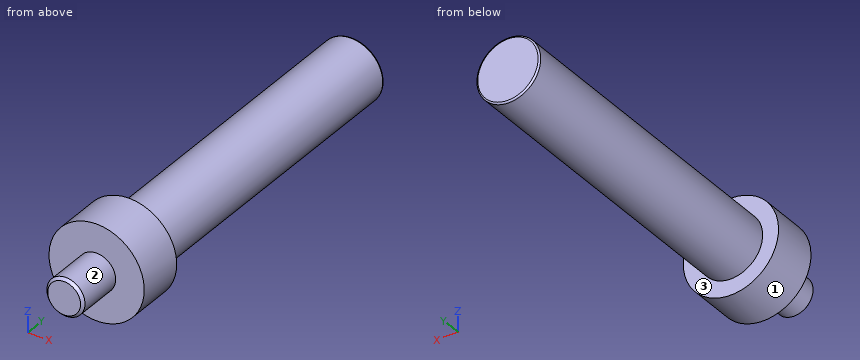
```python
from build123d import *

# Parameters (mm, degrees)
SKETCH1_R           = 15
BOSS_EXTRUDE1_DEPTH = 15
SKETCH2_R           = 10
BOSS_EXTRUDE2_DEPTH = 103
SKETCH3_R           = 7.5
BOSS_EXTRUDE3_DEPTH = 15
FILLET1_R           = 0.5


# Read off the part's stored shape, not the designer's step: M12x1.5 Machine Threads Stud1
with BuildPart() as part:
    # Sketch1 → Boss-Extrude1 (new body)
    with BuildSketch(Plane(origin=(0, 0, 0), x_dir=(1, 0, 0), z_dir=(0, 1, 0))):
        with Locations(Location((0, 0, 0), (0, 0, 270))):
            Circle(SKETCH1_R)
    extrude(amount=BOSS_EXTRUDE1_DEPTH)

    # Sketch2 → Boss-Extrude2 (add)
    with BuildSketch(Plane(origin=(0, 15, 0), x_dir=(1, 0, 0), z_dir=(0, 1, 0))):
        with Locations(Location((0, 0, 0), (0, 0, 270))):
            Circle(SKETCH2_R)
    extrude(amount=BOSS_EXTRUDE2_DEPTH)

    # Sketch3 → Boss-Extrude3 (add)
    with BuildSketch(Plane.XZ):
        with Locations(Location((0, 0, 0), (0, 0, 270))):
            Circle(SKETCH3_R)
    extrude(amount=BOSS_EXTRUDE3_DEPTH)

    # M12x1.5 Machine Threads Stud1 outline → M12x1.5 Machine Threads Stud1 (revolve, cut)
    with BuildSketch(Plane.XY):
        Polygon((7.5, 0), (6, 0), (6, -14.172), (5.172, -15), (7.5, -15), align=None)
    revolve(axis=Axis((0, 0, 0), (0, 1, 0)), mode=Mode.SUBTRACT)

    # Fillet1
    fillet1_edges = [part.edges().sort_by_distance(p)[0] for p in [
        (0, 118, -10),
    ]]
    fillet(fillet1_edges, radius=FILLET1_R)


solid = part.part
```
Build history of the part. All positions in model axes, mm. Face numbers are marked on the shaded views. A direction names the side the tool comes from. Round coordinates to 2 decimals unless told otherwise and drop trailing zeros. Loops run counter-clockwise (first coordinate to the right, second up) from the corner with the lowest first, then second, coordinate; pieces in that order, holes last. Notation, with made-up numbers: M 68.25,56.25 L 91.25,56.25 A29 ccw 91.25,87.25 Z; hole C -31.5,54 d10. An arc over 180 degrees is marked long. Answer as CSV lines item,"result".
1. Flat gauge pins, fed straight in: P1, Ø8, axis at x = -10.5, z = 0.5, coming from the -Y side; P2, Ø2, axis at x = -1.5, y = 30, coming from the -Z side; P3, Ø1.5, axis at y = 16.5, z = 5.5, coming from the +X side. Where does each tip first touch, or does it go through?
Resolved:
P1,"stops at y = 0"
P2,"stops at z = -9.99"
P3,"stops at x = 8.8"
2. Cut at B-B on x = 0. Write the cut outline in (y, z).
Resolved:
outline,"M -15,-5.17 L -14.17,-6 L 0,-6 L 0,-15 L 15,-15 L 15,-10 L 117.5,-10 A0.5 ccw 118,-9.5 L 118,9.5 A0.5 ccw 117.5,10 L 15,10 L 15,15 L 0,15 L 0,6 L -14.17,6 L -15,5.17 Z"
3. 3-axis set-ups, long thin cutter, end or side, ignore diameter. For the marked faces 1, 2 and 3: which of +Z, -Z, +X, -X, +Y, -Y reach the whole face in a straight line?
Resolved:
face 1,"+Y, -Y"
face 2,"-Y"
face 3,"+Y"
4. Cut at A-A on z = 0. Write the cut outline in (x, y).
Resolved:
outline,"M -15,0 L -6,0 L -6,-14.17 L -5.17,-15 L 5.17,-15 L 6,-14.17 L 6,0 L 15,0 L 15,15 L 10,15 L 10,117.5 A0.5 ccw 9.5,118 L -9.5,118 A0.5 ccw -10,117.5 L -10,15 L -15,15 Z"
5. Wall check: probe 1 along Y at (x, z) = (8.5, 11.5); probe 2 along X at (y, z) = (43, 0.75); probe 3 along Y at (x, z) = (-6.25, 5.25). Give the ranges that are in metal, low to high. Write a range as [from, to].
Resolved:
probe 1,"y = [0, 15]"
probe 2,"x = [-9.97, 9.97]"
probe 3,"y = [0, 118]"
6. Cut at C-C on y = 57.5. Write the cut outline in (x, z).
Resolved:
outline,"C 0,0 d20"
7. Cut at D-D on y = -3. Write the cut outline in (x, z), then the cut area to 3 significant figures.
Resolved:
outline,"C 0,0 d12"
area,"113 mm²"
